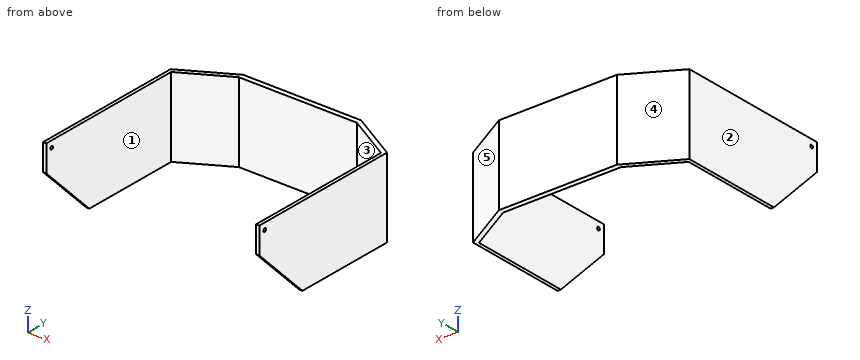
from build123d import *

# Parameters (mm, degrees)
BOSS_EXTRUDE2_DEPTH     = 120
CUT_EXTRUDE2_DEPTH      = 421.861022191
CUT_EXTRUDE2_DEPTH_BACK = 421.861022191
SKETCH5_R               = 2.5


with BuildPart() as part:
    # Sketch3 → Boss-Extrude2 (new body)
    with BuildSketch(Plane.XY):
        Polygon((-5, 5), (-5, -232), (0, -232), (0, 0), (70, 40.414518843), (250, 40.414518843), (320, 0), (320, -232), (325, -232), (325, 5), (250, 48.301270189), (70, 48.301270189), align=None)
    extrude(amount=BOSS_EXTRUDE2_DEPTH)

    # Sketch5 → Cut-Extrude2 (cut, two sides: drawn at the far end of the back side and taken through both)
    with BuildSketch(Plane(origin=(325, 0, 0), x_dir=(0, 0, -1), z_dir=(1, 0, 0)).offset(-CUT_EXTRUDE2_DEPTH_BACK)):
        with Locations((-110, -222)):
            Circle(SKETCH5_R)
        Polygon((-80, -232), (0, -152), (0, -232), align=None)
    extrude(amount=CUT_EXTRUDE2_DEPTH + CUT_EXTRUDE2_DEPTH_BACK, mode=Mode.SUBTRACT)


solid = part.part
Check sheet for the modelled part. Datum: model origin and axes. Units: mm. Face numbers are marked on the shaded views. A direction names the side the tool comes from. Round coordinates to 2 decimals unless told otherwise and drop trailing zeros. Write each loop counter-clockwise with the first axis right and the second up, starting at its lowest first coordinate (ties: lowest second). Pieces come first, ordered by that corner, then holes. Notation, with made-up numbers: (44, 53.5) - (103, 53.5) arc R21 ccw to (103, 78.5) - close; hole circle Ø9 at (6, 40.5). An arc over 180 degrees is marked (long way). Return JSON: item names as keys, results as strings.
Q1. Cross-section at D-D (z = 12). Record the boundary of the cut face in (x, y).
Returned:
{"outline": "(-5, -164) - (0, -164) - (0, 0) - (70, 40.41) - (250, 40.41) - (320, 0) - (320, -164) - (325, -164) - (325, 5) - (250, 48.3) - (70, 48.3) - (-5, 5) - close"}
Q2. Cross-section at B-B (z = 89). Record the boundary of the cut face in (x, y), then the cut area to 3 significant figures.
Returned:
{"outline": "(-5, -232) - (0, -232) - (0, 0) - (70, 40.41) - (250, 40.41) - (320, 0) - (320, -232) - (325, -232) - (325, 5) - (250, 48.3) - (70, 48.3) - (-5, 5) - close", "area": "4,910 mm²"}
Q3. Depth check by flat-ended pin: P1, Ø4, axis at x = 93.5, z = 17.5, coming from the -Y side. Enter the tip coordinate at first touch or a pass-through.
Returned:
{"P1": "stops at y = 40.41"}
Q4. Cross-section at A-A (y = -189). Record the boundary of the cut face in (x, z), then the cut area to 3 significant figures.
Returned:
{"outline": "(-5, 37) - (0, 37) - (0, 120) - (-5, 120) - close; (320, 37) - (325, 37) - (325, 120) - (320, 120) - close", "area": "830 mm²"}
Q5. Draft check along X on the marked faces 3, 4 and 5. Enter one of: released by +X, released by -X, zero draft, split by the parting line, or undercut.
Returned:
{"face 3": "undercut", "face 4": "released by -X", "face 5": "released by +X"}
Q6. Cross-section at C-C (x = 195). Record the boundary of the cut face in (y, z), then the cut area to 3 significant figures.
Returned:
{"outline": "(40.41, 0) - (48.3, 0) - (48.3, 120) - (40.41, 120) - close", "area": "946 mm²"}
Q7. Scan lines: L1, parallel to Z at x = 321.25, y = -222; L2, parallel to X at y = -24, z = 105; L3, parallel to X at y = 10.5, z = 89.5. Record each from-to range of solid material in increasing order. Write a range as from..to.
Returned:
{"L1": "z = 70..107.5, 112.5..120", "L2": "x = -5..0, 320..325", "L3": "x = 4.53..18.19, 301.81..315.47"}
Q8. Access from +Z, -Z, +X, -X, +Y, -Y to the whole of each face (thin tool, end or side, straight path). Record for the marked faces 1 and 2.
Returned:
{"face 1": "+Z, -Z, -Y", "face 2": "+Z, -Z, -X, +Y, -Y"}
